Could you check a few things on this model? Use its own coordinates, in mm. A direction names the side the tool comes from. Round coordinates to 2 decimals unless told otherwise and drop trailing zeros. Loops run counter-clockwise (first coordinate to the right, second up) from the corner with the lowest first, then second, coordinate; pieces in that order, holes last. Notation, with made-up numbers: (45, -18.75) -> (90, -18.75) arc R5 cw to (90, -14.75) -> close; hole circle Ø9 at (-31, 4.25). An arc over 180 degrees is marked (long way). Write each question's results on one line, items separated by ' | '. Start each with the question number.
1) Imagine slicing it at D-D, the plane z = -10. List the corners of the cut face in (x, y) for me (1 decimal), plus the area to 3 significant figures.
2) Imagine slicing it at A-A, the plane z = -20.5. List the corners of the cut face in (x, y) for me, plus the area to 3 significant figures.
3) We'd pull the mould along X, two halves only. Please class faces 4 (the flat face through (-73.63, -4.85, -13.5)), 5 (the flat face through (-57, 0, -20)), 6 (the flat face through (-39.198, -10, -14)): pulls with the +X half, pulls with the -X half, needs draft (parallel to the pull), parting line crosses it, or undercut.
4) Imagine slicing it at C-C, the plane y = -52.5. List the corners of the cut face in (x, z) for me, plus the area to 3 significant figures.
5) For P1, Ø0.7, axis at x = -74.5, z = -15.5, coming from the -Y side; P2, Ø8, axis at x = -52.5, y = -33, coming from the +Z side; P3, Ø7.5, axis at y = -12, z = -11.5, coming from the -X side, each with a flat end and sliding along its axis, tell me the tip position at first contact or that it passes through.
6) If I drill on probe 1 along Y at (x, z) = (-57, -20.6); probe 2 along Z at (x, y) = (-72, -36.5); probe 3 along X at (y, z) = (-14.5, -12.75), over which ranges is the centre line in solid material (lowest first)?
7) Which directions (+Z, -Z, +X, -X, +Y, -Y) give clear straight access to the entire face, cutting with the end or side of a thin tool? Please do faces 1 (the flat face through (-40.871, -10, -14)), 2 (the cylindrical face through (-67.891, -8.603, -13.502)), 3 (the flat face through (-74.801, -10, -14)).
8) Imagine slicing it at B-B, the plane x = -57. List the corners of the cut face in (y, z) for me, plus the area to 3 significant figures.
from build123d import *

# Parameters (mm, degrees)
BOSS_EXTRUDE1_START = -18.343704
SKETCH1_W           = 40
SKETCH1_H           = 58.259460065
SKETCH1_R           = 5.396381747
BOSS_EXTRUDE1_DEPTH = 3.18
FILLET1_R           = 10
SKETCH2_R           = 1.735008093
SKETCH2_R_2         = 1.656779544
BOSS_EXTRUDE2_DEPTH = 13


with BuildPart() as part:
    # Sketch1 → Boss-Extrude1 (new body)
    with BuildSketch(Plane.XY.offset(BOSS_EXTRUDE1_START)):
        with Locations((-57, -29.129730033)):
            Rectangle(SKETCH1_W, SKETCH1_H)
        with Locations((-57, -49.150000002)):
            Circle(SKETCH1_R, mode=Mode.SUBTRACT)
    extrude(amount=-BOSS_EXTRUDE1_DEPTH)

    # Fillet1
    fillet1_edges = [part.edges().sort_by_distance(p)[0] for p in [
        (-37, -58.259460066, -19.933704),
        (-77, -58.259460066, -19.933704),
    ]]
    fillet(fillet1_edges, radius=FILLET1_R)

    # Sketch2 → Boss-Extrude2 (add)
    with BuildSketch(Plane(origin=(0, 0, -21.523704006), x_dir=(-1, 0, 0), z_dir=(0, 0, -1))):
        with Locations((47.000000001, -10.000000002)):
            Circle(SKETCH2_R)
        with Locations((67.000376739, -10.000360351)):
            Circle(SKETCH2_R_2)
        Polygon((74.800685175, -15.79650853), (74.800685175, -4.278676416), (74.207239255, -4.278676416), (73.035580783, -5.437870437), (73.035580783, -14.663272101), (74.156761506, -15.79650853), align=None)
        Polygon((39.198491865, -15.79650853), (39.198491865, -4.122433506), (39.836367638, -4.122433506), (40.870792952, -5.11185736), (40.870792952, -14.618450275), (39.807051778, -15.79650853), align=None)
    extrude(amount=-BOSS_EXTRUDE2_DEPTH)


solid = part.part
Checked values:
1) outline: (-74.8, -15.8) -> (-74.2, -15.8) -> (-73, -14.7) -> (-73, -5.4) -> (-74.2, -4.3) -> (-74.8, -4.3) -> close; circle Ø3.3 at (-67, -10); circle Ø3.5 at (-47, -10); (-40.9, -14.6) -> (-39.8, -15.8) -> (-39.2, -15.8) -> (-39.2, -4.1) -> (-39.8, -4.1) -> (-40.9, -5.1) -> close | area: 55.5 mm^2
2) outline: (-77, -48.26) arc R10 ccw to (-67, -58.26) -> (-47, -58.26) arc R10 ccw to (-37, -48.26) -> (-37, 0) -> (-77, 0) -> close; hole circle Ø10.79 at (-57, -49.15) | area: 2,200 mm^2
3) face 4: undercut | face 5: needs draft | face 6: pulls with the +X half
4) outline: (-76.06, -21.52) -> (-61.23, -21.52) -> (-61.23, -18.34) -> (-76.06, -18.34) -> close; (-52.77, -21.52) -> (-37.94, -21.52) -> (-37.94, -18.34) -> (-52.77, -18.34) -> close | area: 94.3 mm^2
5) P1: y = -15.8 | P2: z = -18.34 | P3: x = -74.8
6) probe 1: -58.26 to -54.55, -43.75 to 0 | probe 2: -21.52 to -18.34 | probe 3: -74.8 to -73.04, -40.87 to -39.2
7) face 1: +Z, +Y, -Y | face 2: +Z | face 3: +Z, -X, +Y, -Y
8) outline: (-58.26, -21.52) -> (-54.55, -21.52) -> (-54.55, -18.34) -> (-58.26, -18.34) -> close; (-43.75, -21.52) -> (0, -21.52) -> (0, -18.34) -> (-43.75, -18.34) -> close | area: 151 mm^2
